from build123d import *

# Parameters (mm, degrees)
SKETCH2_R               = 2.25
BOSS_EXTRUDE1_DEPTH     = 3.175
SKETCH1_W               = 2.16
SKETCH1_H               = 4.8
SKETCH1_H_2             = 25.4
SKETCH1_W_2             = 57.84
SKETCH1_R               = 1.63
BOSS_EXTRUDE2_DEPTH     = 3.175
TOP_CONNECTION_SKETCH_W = 35
TOP_CONNECTION_SKETCH_H = 3.175
CHAMFER1_SIZE           = 4.8
CHAMFER2_SIZE           = 0.41
CHAMFER2_SIZE_2         = 0.434896144


# Some blends are built 0.0001 mm under size
with BuildPart() as part:
    # Sketch2 → Boss-Extrude1 (new body)
    with BuildSketch(Plane(origin=(0, 87.18, 0), x_dir=(1, 0, 0), z_dir=(0, 1, 0))):
        with BuildLine():
            ThreePointArc((38.5, 0), (27.3118564, 27.135078773), (0.25, 38.499188303))
            Line((0.25, 38.499188303), (0.25, 26.248809497))
            ThreePointArc((0.25, 26.248809497), (18.649731902, 18.472953202), (26.25, 0))
            ThreePointArc((26.25, 0), (18.649731902, -18.472953202), (0.25, -26.248809497))
            Line((0.25, -26.248809497), (0.25, -38.499188303))
            ThreePointArc((0.25, -38.499188303), (27.3118564, -27.135078773), (38.5, 0))
        make_face()
        with Locations(Location((12.819894984, -30.949964339, 0), (0, 0, 270))):
            Circle(SKETCH2_R, mode=Mode.SUBTRACT)
        with Locations(Location((30.949964339, -12.819894984, 0), (0, 0, 270))):
            Circle(SKETCH2_R, mode=Mode.SUBTRACT)
        with Locations(Location((30.949964339, 12.819894984, 0), (0, 0, 270))):
            Circle(SKETCH2_R, mode=Mode.SUBTRACT)
        with Locations(Location((12.819894984, 30.949964339, 0), (0, 0, 270))):
            Circle(SKETCH2_R, mode=Mode.SUBTRACT)
    extrude(amount=-BOSS_EXTRUDE1_DEPTH)



with BuildPart() as body_2:
    # Sketch1 → Boss-Extrude2 (new body)
    # profile 1 of 4: a face of its own
    with BuildSketch(Plane(origin=(0, 0, 0), x_dir=(1, 0, 0), z_dir=(0, 1, 0))):
        with Locations((78.92, 15.1)):
            Rectangle(SKETCH1_W, SKETCH1_H)
    # profile 2 of 4: a face of its own
    with BuildSketch(Plane(origin=(0, 0, 0), x_dir=(1, 0, 0), z_dir=(0, 1, 0))):
        with Locations((78.92, 0)):
            Rectangle(SKETCH1_W, SKETCH1_H_2)
    # profile 3 of 4: a face of its own
    with BuildSketch(Plane(origin=(0, 0, 0), x_dir=(1, 0, 0), z_dir=(0, 1, 0))):
        with Locations((48.92, 0)):
            Rectangle(SKETCH1_W_2, SKETCH1_H_2)
        with Locations(Location((26.35, -6.35, 0), (0, 0, 270))):
            Circle(SKETCH1_R, mode=Mode.SUBTRACT)
        with Locations(Location((41.35, -6.35, 0), (0, 0, 270))):
            Circle(SKETCH1_R, mode=Mode.SUBTRACT)
        with Locations(Location((56.35, -6.35, 0), (0, 0, 270))):
            Circle(SKETCH1_R, mode=Mode.SUBTRACT)
        with Locations(Location((71.35, -6.35, 0), (0, 0, 270))):
            Circle(SKETCH1_R, mode=Mode.SUBTRACT)
        with Locations(Location((26.35, 6.35, 0), (0, 0, 270))):
            Circle(SKETCH1_R, mode=Mode.SUBTRACT)
        with Locations(Location((41.35, 6.35, 0), (0, 0, 270))):
            Circle(SKETCH1_R, mode=Mode.SUBTRACT)
        with Locations(Location((56.35, 6.35, 0), (0, 0, 270))):
            Circle(SKETCH1_R, mode=Mode.SUBTRACT)
        with Locations(Location((71.35, 6.35, 0), (0, 0, 270))):
            Circle(SKETCH1_R, mode=Mode.SUBTRACT)
    # profile 4 of 4: a face of its own
    with BuildSketch(Plane(origin=(0, 0, 0), x_dir=(1, 0, 0), z_dir=(0, 1, 0))):
        with Locations((78.92, -15.1)):
            Rectangle(SKETCH1_W, SKETCH1_H)
    extrude(amount=BOSS_EXTRUDE2_DEPTH)


with BuildPart() as part_1:
    add(part.part)

    add(body_2.part)  # Sweep2 merges body 2
    # Sweep2: sweep along a curve in space
    with BuildLine() as sweep2_path:
        ThreePointArc((80.58, 0, 17.5), (83.80445923, 57.472384507, 17.5), (34.5, 87.18, 17.5))
    # Top_Connection_Sketch → Sweep2 (sweep)
    with BuildSketch(Plane(origin=(34.5, 0, 0), x_dir=(0, 0, -1), z_dir=(1, 0, 0))):
        with Locations((0, 85.5925)):
            Rectangle(TOP_CONNECTION_SKETCH_W, TOP_CONNECTION_SKETCH_H)
    sweep(path=sweep2_path.line)

    # Chamfer1
    chamfer1_edges = [part_1.edges().sort_by_distance(p)[0] for p in [
        (77.84, 1.5875, -12.7),
        (77.84, 1.5875, 12.7),
    ]]
    chamfer(chamfer1_edges, length=CHAMFER1_SIZE - 0.0001)  # a hair under: the kernel refuses the full size

    # Chamfer2
    # the kernel refuses this chamfer: 0.434896144, 0.41 mm, written as the material it adds along each edge
    with BuildSketch(Plane(origin=(34.5, 84.005, 17.088007491), x_dir=(0.04194571569864223, 0, 0.9991198911714894), z_dir=(0, 1, 0))) as chamfer2_piece_1:
        with BuildLine():
            Line((CHAMFER2_SIZE * 0.999119891171, -CHAMFER2_SIZE * 0.0419457156986), (CHAMFER2_SIZE_2 * 0.873966952265, -CHAMFER2_SIZE_2 * 0.485985357052))
            ThreePointArc((CHAMFER2_SIZE_2 * 0.873966952265, -CHAMFER2_SIZE_2 * 0.485985357052), (0.192993875, -0.106615288), (0, 0))
            Line((0, 0), (CHAMFER2_SIZE * 0.999119891171, -CHAMFER2_SIZE * 0.0419457156986))
        make_face()
    extrude(amount=3.175)


solid = part_1.part
Here's how the part is built. I have some questions about the finished solid (model axes, mm). A direction names the side the tool comes from. Coordinates: 2 decimals unless noted, no trailing zeros. Write each loop counter-clockwise with the first axis right and the second up, starting at its lowest first coordinate (ties: lowest second). Pieces come first, ordered by that corner, then holes. Notation, with made-up numbers: (8.25, 15.5) - (53.25, 15.5) arc R32 cw to (53.25, 51.5) - close; hole circle Ø7 at (-16.75, 44.5). An arc over 180 degrees is marked (long way). Use one line per item in the form item = value.
1) Suppose I cut it at D-D, the plane y = 20.5. Write out the boundary of the cut face in (x, z), plus the area to 3 significant figures.
Solved:
outline = (85.95, -17.5) - (89.19, -17.5) - (89.19, 17.5) - (85.95, 17.5) - close
area = 113 mm2
2) On a 3-axis mill with a long thin cutter (end or side, diameter ignored), from which of +Z, -Z, +X, -X, +Y, -Y can I reach the whole of each face in a straight line? I mean faces 4 (the flat face through (49, 3.175, 0)), 5 (the cylindrical face through (72.966, 1.565, 6.138)), 6 (the flat face through (75.41, 1.57, 15.07)). Say none if no direction works.
Solved:
face_4 = +Z, -Z, -X
face_5 = -Y
face_6 = +Z, -X, -Y
3) I need wall thicknesses on line 1 (X direction, y = 2, z = 6); line 2 (X direction, y = 2.5, z = 6.35); line 3 (Y direction, x = 13.5, z = 23.5) (3 decimals). Which ranges of each line are inside material? Lowest first, please.
Solved:
line_1 = 20 to 24.76, 27.94 to 39.76, 42.94 to 54.76, 57.94 to 69.76, 72.94 to 81.88
line_2 = 20 to 24.72, 27.98 to 39.72, 42.98 to 54.72, 57.98 to 69.72, 72.98 to 82.19
line_3 = 84.005 to 87.18
4) Suppose I cut it at B-B, the plane x = 68.5. Write out the boundary of the cut face in (y, z) (3 decimals), plus the area to 3 significant figures.
Solved:
outline = (0, -12.7) - (3.175, -12.7) - (3.175, 12.7) - (0, 12.7) - close; (71.537, -17.5) - (75.617, -17.5) - (75.617, 17.5) - (71.537, 17.5) - close
area = 223 mm2
5) Suppose I cut it at C-C, the plane x = 56.35. Write out the boundary of the cut face in (y, z) (3 decimals), plus the area to 3 significant figures.
Solved:
outline = (0, -12.7) - (3.175, -12.7) - (3.175, -7.98) - (0, -7.98) - close; (0, -4.72) - (3.175, -4.72) - (3.175, 4.72) - (0, 4.72) - close; (0, 7.98) - (3.175, 7.98) - (3.175, 12.7) - (0, 12.7) - close; (79.251, -17.5) - (82.721, -17.5) - (82.721, 17.5) - (79.251, 17.5) - close
area = 181 mm2
6) I'm going to push flat-ended pins straight in: P1, Ø3, axis at y = 23.5, z = -8.5, coming from the +X side; P2, Ø10, axis at y = 44, z = -9, coming from the -X side (3 decimals); P3, Ø8, axis at y = 45, z = 21, coming from the -X side; P4, Ø5, axis at x = 26.35, z = -6.35, coming from the -Y side. Where does each tip first touch, or does it pass through?
Solved:
P1 = 89.9
P2 = 84.065
P3 = 84.75
P4 = 0
7) Suppose I cut it at A-A, the plane z = 6.35. Write out the boundary of the cut face in (x, y) (3 decimals).
Solved:
outline = (20, 0) - (24.72, 0) - (24.72, 3.175) - (20, 3.175) - close; (25.47, 84.005) - (34.5, 84.005) arc R52.593 cw to (78.87, 3.175) - (72.98, 3.175) - (72.98, 0) - (80, 0) - (80, 0.395) - (80.58, 0) arc R55.768 ccw to (37.973, 87.072) - (37.973, 87.18) - (25.47, 87.18) - close; (27.98, 0) - (39.72, 0) - (39.72, 3.175) - (27.98, 3.175) - close; (42.98, 0) - (54.72, 0) - (54.72, 3.175) - (42.98, 3.175) - close; (57.98, 0) - (69.72, 0) - (69.72, 3.175) - (57.98, 3.175) - close
8) Thinking about a two-plate mould opening in X: for faces 1 (the flat face through (83, 53, 17.5)), 2 (the cylindrical face through (28.954, 85.615, -11.782)), 3 (the cylindrical face through (84.194, 56.721, 0.245)), which applies, released by +X, released by -X, zero draft, split by the parting line, or undercut?
Solved:
face_1 = zero draft
face_2 = undercut
face_3 = released by +X
